Source: CAD feature listing. Evaluate the final solid. Frame: model axes, mm. Face numbers are marked on the shaded views. A direction names the side the tool comes from. Give positions to 0.01 mm unless a question says otherwise; leave off trailing zeros. Loops run counter-clockwise (first coordinate to the right, second up) from the corner with the lowest first, then second, coordinate; pieces in that order, holes last. Notation, with made-up numbers: M 16,47 L 20,47 A24 ccw 20,67 Z; hole C -2.75,39.25 d4. An arc over 180 degrees is marked long. Answer in a Markdown table with one row per item.
```python
from build123d import *

# Parameters (mm, degrees)
ESQUISSE1_W        = 42
ESQUISSE1_H        = 24
ESQUISSE1_R        = 9.75
ESQUISSE1_R_2      = 4.75
BOSS_EXTRU_2_DEPTH = 2.5
ESQUISSE3_W        = 3
ESQUISSE3_H        = 24
BOSS_EXTRU_5_DEPTH = 7.5
BOSS_EXTRU_6_DEPTH = 3
ESQUISSE7_W        = 24
ESQUISSE7_H        = 2.5
BOSS_EXTRU_7_DEPTH = 3


with BuildPart() as part:
    # Esquisse1 → Boss.-Extru.2 (new body)
    # profile 1 of 3: a face of its own
    with BuildSketch(Plane(origin=(0, 0, 0), x_dir=(1, 0, 0), z_dir=(0, 1, 0))):
        with Locations((21, 12)):
            Rectangle(ESQUISSE1_W, ESQUISSE1_H)
        with Locations((21, 12)):
            Circle(ESQUISSE1_R, mode=Mode.SUBTRACT)
    # profile 2 of 3: a face of its own
    with BuildSketch(Plane(origin=(0, 0, 0), x_dir=(1, 0, 0), z_dir=(0, 1, 0))):
        with Locations((21, 12)):
            Circle(ESQUISSE1_R)
        with Locations((21, 12)):
            Circle(ESQUISSE1_R_2, mode=Mode.SUBTRACT)
    # profile 3 of 3: a face of its own
    with BuildSketch(Plane(origin=(0, 0, 0), x_dir=(1, 0, 0), z_dir=(0, 1, 0))):
        with Locations((21, 12)):
            Circle(ESQUISSE1_R_2)
    extrude(amount=BOSS_EXTRU_2_DEPTH)

    # Esquisse3 → Boss.-Extru.5 (add)
    with BuildSketch(Plane.XZ):
        Polygon((42, 0), (44.999473272, -0.056214692), (45, -24.056214686), (42, -24.056214686), align=None)
        with Locations((-1.5, -12)):
            Rectangle(ESQUISSE3_W, ESQUISSE3_H)
    extrude(amount=-BOSS_EXTRU_5_DEPTH)

    # Esquisse6 → Boss.-Extru.6 (add)
    with BuildSketch(Plane.ZY.offset(-42)):
        Polygon((-24.056214686, 4.962472786), (0, 5), (0, 7.5), (-24.056214686, 7.5), align=None)
    extrude(amount=BOSS_EXTRU_6_DEPTH)

    # Esquisse7 → Boss.-Extru.7 (add)
    with BuildSketch(Plane(origin=(0, 0, 0), x_dir=(0, 0, -1), z_dir=(1, 0, 0))):
        with Locations((12, 6.25)):
            Rectangle(ESQUISSE7_W, ESQUISSE7_H)
    extrude(amount=BOSS_EXTRU_7_DEPTH)


solid = part.part
```
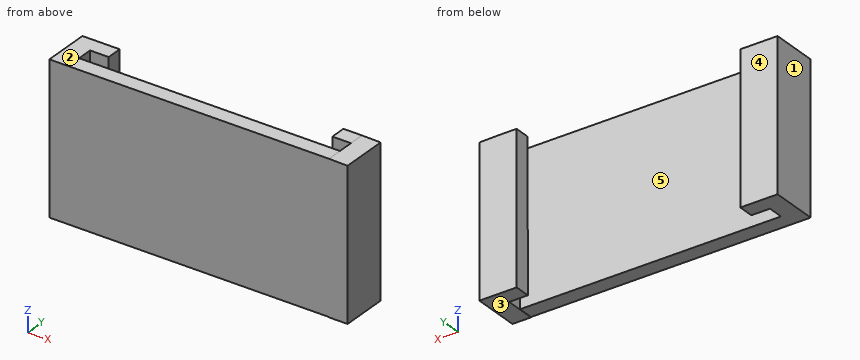
1) Pin query (flat end, axial travel): pin 1 Ø12 at (x, z) = (17.5, -11) entering from +Y; pin 2 Ø1 at (x, y) = (37, 5) entering from +Z; pin 3 Ø4 at (x, y) = (29.5, 2) entering from -Z. Return the tip coordinate at first contact, or that it passes through.
Reply:
| item | result |
|---|---|
| pin 1 | stops at y = 2.5 |
| pin 2 | passes through |
| pin 3 | stops at z = -24 |
2) Section A-A, the plane y = 4.25. Return loops of the section in (x, z), then the cut area to 3 significant figures.
Reply:
| item | result |
|---|---|
| outline | M -3,-24 L 0,-24 L 0,0 L -3,0 Z; M 42,-24.06 L 45,-24.06 L 45,-0.06 L 42,0 Z |
| area | 144 mm² |
3) Section D-D, the plane x = 36. Return loops of the section in (y, z), then the cut area to 3 significant figures.
Reply:
| item | result |
|---|---|
| outline | M 0,-24 L 2.5,-24 L 2.5,0 L 0,0 Z |
| area | 60.0 mm² |
4) Section C-C, the plane z = -11. Return loops of the section in (x, y), then the cut area to 3 significant figures.
Reply:
| item | result |
|---|---|
| outline | M -3,0 L 45,0 L 45,7.5 L 39,7.5 L 39,4.98 L 42,4.98 L 42,2.5 L 0,2.5 L 0,5 L 3,5 L 3,7.5 L -3,7.5 Z |
| area | 165 mm² |
5) Pull-direction query (Z, two-part tool) for the marked faces 1, 2 and 3; classes: released by +Z, released by -Z, zero draft, split by the parting line, or undercut.
Reply:
| item | result |
|---|---|
| face 1 | zero draft |
| face 2 | released by +Z |
| face 3 | released by -Z |
6) Section B-B, the plane x = 2.5. Return loops of the section in (y, z).
Reply:
| item | result |
|---|---|
| outline | M 0,-24 L 2.5,-24 L 2.5,0 L 0,0 Z; M 5,-24 L 7.5,-24 L 7.5,0 L 5,0 Z |
7) Material intervals for L1, parallel to Y at x = 1, z = -19.5; L2, parallel to X at y = 5.75, z = -11; L3, parallel to X at y = 4.25, z = -11.5, sorted ascending.
Reply:
| item | result |
|---|---|
| L1 | y = 0 to 2.5, 5 to 7.5 |
| L2 | x = -3 to 3, 39 to 45 |
| L3 | x = -3 to 0, 42 to 45 |
8) Set-up query: the marked faces 4 and 5. Return all of +Z, -Z, +X, -X, +Y, -Y with unobstructed straight access to the full face (end or side cutting, diameter ignored); none if empty.
Reply:
| item | result |
|---|---|
| face 4 | +Z, -Z, +X, -X, +Y |
| face 5 | +Z, -Z |
